Model file for the job. Use its own axes, mm. Face numbers are marked on the shaded views. A direction names the side the tool comes from. Round coordinates to 2 decimals unless told otherwise and drop trailing zeros. Loops run counter-clockwise (first coordinate to the right, second up) from the corner with the lowest first, then second, coordinate; pieces in that order, holes last. Notation, with made-up numbers: (-22.5, -25) -> (4.5, -25) arc R22 cw to (4.5, 2) -> close; hole circle Ø8 at (53, 79.5). An arc over 180 degrees is marked (long way). Use a Markdown table: item, result.
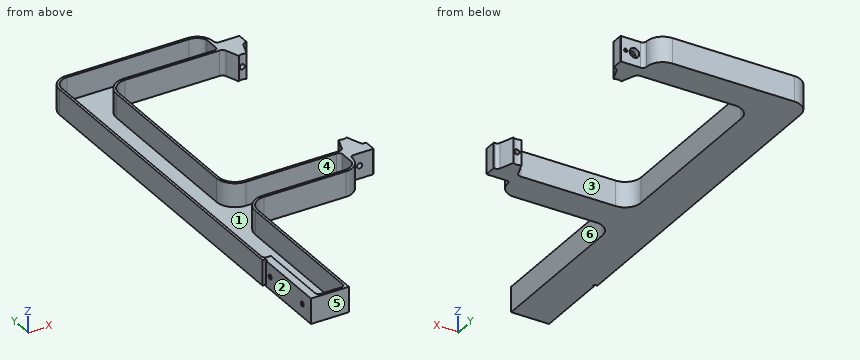
from build123d import *

# Parameters (mm, degrees)
BOSS_EXTRUDE1_DEPTH              = 15.875
SKETCH13_W                       = 2.54
SKETCH13_H                       = 95.25
CUT_EXTRUDE2_DEPTH               = 32.75
SKETCH14_W                       = 1.6002
SKETCH14_H                       = 3.302
CUT_EXTRUDE3_DEPTH               = 32.75
FILLET4_R                        = 1.5875
FILLET1_R                        = 6.35
FILLET2_R                        = 20
FILLET3_R                        = 4.7625
SKETCH10_R                       = 6
CUT_EXTRUDE1_DEPTH               = 7
F_4_40_TAPPED_HOLE1_D            = 2.2606
F_4_40_TAPPED_HOLE1_DEPTH        = 7.6
F_4_40_TAPPED_HOLE1_CSINK_D      = 4.1148
F_4_40_TAPPED_HOLE1_CSINK_ANGLE  = 90
F_4_40_TAPPED_HOLE1_TIP          = 0.679152758
CHAMFER1_SIZE                    = 0.5
F_10_32_TAPPED_HOLE1_D           = 4.0386
F_10_32_TAPPED_HOLE1_DEPTH       = 12.03
F_10_32_TAPPED_HOLE1_CSINK_D     = 6.096
F_10_32_TAPPED_HOLE1_CSINK_ANGLE = 90
F_10_32_TAPPED_HOLE1_TIP         = 1.213317848
CUT_EXTRUDE7_DEPTH               = 29.75
FILLET5_R                        = 4.7625


with BuildPart() as part:
    # Sketch1 → Boss-Extrude1 (new body, symmetric)
    with BuildSketch(Plane.XY):
        with BuildLine():
            Line((-313, -123), (-176.364963641, -123))
            Line((-176.364963641, -123), (-170.374987965, -123))
            Line((-170.374987965, -123), (-162.97678843, -102.673613833))
            ThreePointArc((-162.97678843, -102.673613833), (-158, -104), (-153.02321157, -102.673613833))
            Line((-153.02321157, -102.673613833), (-145.625012035, -123))
            Line((-145.625012035, -123), (-140.625012035, -123))
            Line((-140.625012035, -123), (-140.625012035, -138))
            Line((-140.625012035, -138), (-145.625012035, -138))
            Line((-145.625012035, -138), (-170.374987965, -138))
            Line((-170.374987965, -138), (-170.374987965, -163))
            Line((-170.374987965, -163), (-313, -163))
            Line((-313, -163), (-313, -370.4))
            Line((-313, -370.4), (-363, -370.4))
            Line((-363, -370.4), (-363, -163))
            Line((-363, -163), (-363, 163))
            Line((-363, 163), (-170.374987965, 163))
            Line((-170.374987965, 163), (-170.374987965, 138))
            Line((-170.374987965, 138), (-145.625012035, 138))
            Line((-145.625012035, 138), (-140.625012035, 138))
            Line((-140.625012035, 138), (-140.625012035, 123))
            Line((-140.625012035, 123), (-145.625012035, 123))
            Line((-145.625012035, 123), (-153.02321157, 102.673613833))
            ThreePointArc((-153.02321157, 102.673613833), (-158, 104), (-162.97678843, 102.673613833))
            Line((-162.97678843, 102.673613833), (-170.374987965, 123))
            Line((-170.374987965, 123), (-176.364963641, 123))
            Line((-176.364963641, 123), (-313, 123))
            Line((-313, 123), (-313, -123))
        make_face()
    extrude(amount=BOSS_EXTRUDE1_DEPTH, both=True)

    # Sketch13 → Cut-Extrude2 (cut, through all)
    with BuildSketch(Plane.XY.offset(15.875)):
        with Locations((-361.73, -322.775)):
            Rectangle(SKETCH13_W, SKETCH13_H)
    extrude(amount=-CUT_EXTRUDE2_DEPTH, mode=Mode.SUBTRACT)

    # Sketch14 → Cut-Extrude3 (cut, through all)
    with BuildSketch(Plane.XY.offset(15.875)):
        with Locations((-359.6599, -276.801)):
            Rectangle(SKETCH14_W, SKETCH14_H)
    extrude(amount=-CUT_EXTRUDE3_DEPTH, mode=Mode.SUBTRACT)

    # Fillet4
    fillet4_edges = [part.edges().sort_by_distance(p)[0] for p in [
        (-358.8598, -275.15, 0),
        (-358.8598, -278.452, 0),
    ]]
    fillet(fillet4_edges, radius=FILLET4_R)

    # Fillet1
    fillet1_edges = [part.edges().sort_by_distance(p)[0] for p in [
        (-170.374987965, -123, 0),
        (-170.374987965, 123, 0),
    ]]
    fillet(fillet1_edges, radius=FILLET1_R)

    # Fillet2
    fillet2_edges = [part.edges().sort_by_distance(p)[0] for p in [
        (-313, 123, 0),
        (-313, -123, 0),
        (-170.374987965, -163, 0),
        (-313, -163, 0),
        (-363, 163, 0),
        (-170.374987965, 163, 0),
    ]]
    fillet(fillet2_edges, radius=FILLET2_R)

    # Fillet3
    fillet3_edges = [part.edges().sort_by_distance(p)[0] for p in [
        (-145.625012035, -123, 0),
        (-170.374987965, -138, 0),
        (-170.374987965, 138, 0),
        (-145.625012035, 123, 0),
    ]]
    fillet(fillet3_edges, radius=FILLET3_R)

    # Sketch8 → M6 Clearance Hole1 (revolve, cut)
    with BuildSketch(Plane(origin=(-158, 138, 0), x_dir=(0, 0, 1), z_dir=(1, 0, 0))):
        Polygon((0, 0), (0, 51.960753981), (3.2, 50.038), (3.2, 0), align=None)
    m6_clearance_hole1 = revolve(axis=Axis((-158, 144.35, 0), (0, -1, 0)), mode=Mode.SUBTRACT)

    # Sketch10 → Cut-Extrude1 (cut)
    with BuildSketch(Plane(origin=(0, 138, 0), x_dir=(1, 0, 0), z_dir=(0, 1, 0))):
        with Locations(Location((-158, 0, 0), (0, 0, 270))):  # turned: the seam where the file's is
            Circle(SKETCH10_R)
    extrude(amount=-CUT_EXTRUDE1_DEPTH, mode=Mode.SUBTRACT)

    # #4-40 Tapped Hole1
    with Locations(Plane(origin=(0, 138, 0), x_dir=(-1, 0, 0), z_dir=(0, 1, 0))):
        with Locations((147, 0)):
            CounterSinkHole(F_4_40_TAPPED_HOLE1_D / 2, F_4_40_TAPPED_HOLE1_CSINK_D / 2, depth=F_4_40_TAPPED_HOLE1_DEPTH, counter_sink_angle=F_4_40_TAPPED_HOLE1_CSINK_ANGLE)
            with Locations((0, 0, -(F_4_40_TAPPED_HOLE1_DEPTH + F_4_40_TAPPED_HOLE1_TIP / 2))):  # 118° drill point
                Cone(0, F_4_40_TAPPED_HOLE1_D / 2, F_4_40_TAPPED_HOLE1_TIP, mode=Mode.SUBTRACT)

    # Mirror1: M6 Clearance Hole1 across plane
    add(m6_clearance_hole1.mirror(Plane.ZX), mode=Mode.SUBTRACT)

    # Chamfer1
    chamfer1_edges = [part.edges().sort_by_distance(p)[0] for p in [
        (-140.625012035, -138, 0),
        (-140.625012035, 138, 0),
    ]]
    chamfer(chamfer1_edges, length=CHAMFER1_SIZE)

    # #10-32 Tapped Hole1
    with Locations(Plane.ZY.offset(360.46)):
        with Locations((0, -286.58), (0, -352.62)):
            CounterSinkHole(F_10_32_TAPPED_HOLE1_D / 2, F_10_32_TAPPED_HOLE1_CSINK_D / 2, depth=F_10_32_TAPPED_HOLE1_DEPTH, counter_sink_angle=F_10_32_TAPPED_HOLE1_CSINK_ANGLE)
            with Locations((0, 0, -(F_10_32_TAPPED_HOLE1_DEPTH + F_10_32_TAPPED_HOLE1_TIP / 2))):  # 118° drill point
                Cone(0, F_10_32_TAPPED_HOLE1_D / 2, F_10_32_TAPPED_HOLE1_TIP, mode=Mode.SUBTRACT)

    # Sketch25 → Cut-Extrude7 (cut)
    with BuildSketch(Plane.XY.offset(15.875)):
        with BuildLine():
            Line((-190.374987965, 160), (-343, 160))
            ThreePointArc((-343, 160), (-355.02081528, 155.02081528), (-360, 143))
            Line((-360, 143), (-360, -272.15))
            Line((-360, -272.15), (-350.808, -272.15))
            Line((-350.808, -272.15), (-350.808, -367.4))
            Line((-350.808, -367.4), (-316, -367.4))
            Line((-316, -367.4), (-316, -183))
            ThreePointArc((-316, -183), (-309.263455967, -166.736544033), (-293, -160))
            Line((-293, -160), (-190.374987965, -160))
            ThreePointArc((-190.374987965, -160), (-181.091910782, -157.241645903), (-174.821305833, -149.861703296))
            Line((-174.821305833, -149.861703296), (-174.821305833, -126))
            Line((-174.821305833, -126), (-293, -126))
            ThreePointArc((-293, -126), (-309.263455967, -119.263455967), (-316, -103))
            Line((-316, -103), (-316, 103))
            ThreePointArc((-316, 103), (-309.263455967, 119.263455967), (-293, 126))
            Line((-293, 126), (-174.821305833, 126))
            Line((-174.821305833, 126), (-174.821305833, 149.861703296))
            ThreePointArc((-174.821305833, 149.861703296), (-181.091910782, 157.241645903), (-190.374987965, 160))
        make_face()
    extrude(amount=-CUT_EXTRUDE7_DEPTH, mode=Mode.SUBTRACT)

    # Fillet5
    fillet5_edges = [part.edges().sort_by_distance(p)[0] for p in [
        (-350.808, -367.4, 1),
        (-316, -367.4, 1),
        (-174.821305833, -149.861703296, 1),
        (-174.821305833, -126, 1),
        (-174.821305833, 126, 1),
        (-174.821305833, 149.861703296, 1),
        (-360, -272.15, 1),
    ]]
    fillet(fillet5_edges, radius=FILLET5_R)


solid = part.part
Q1. Pull direction Y, two halves, no side cores. Call the marked faces 4, 5 and 6: released by +Y, released by -Y, zero draft, split by the parting line, or undercut.
Results list:
| item | result |
|---|---|
| face 4 | undercut |
| face 5 | released by -Y |
| face 6 | zero draft |
Q2. Band-saw the part on C-C, the plane x = -329. Give the cut face in (y, z) (3 decimals), plus the area to 3 significant figures.
Results list:
| item | result |
|---|---|
| outline | (-370.4, -15.875) -> (163, -15.875) -> (163, 15.875) -> (160, 15.875) -> (160, -13.875) -> (-367.4, -13.875) -> (-367.4, 15.875) -> (-370.4, 15.875) -> close |
| area | 1,250 mm² |
Q3. Band-saw the part on B-B, the plane y = -69.5. Give the cut face in (x, z) (3 decimals), plus the area to 4 significant figures.
Results list:
| item | result |
|---|---|
| outline | (-363, -15.875) -> (-313, -15.875) -> (-313, 15.875) -> (-316, 15.875) -> (-316, -13.875) -> (-360, -13.875) -> (-360, 15.875) -> (-363, 15.875) -> close |
| area | 278.5 mm² |
Q4. Band-saw the part on A-A, the plane x = -196.5. Give the cut face in (y, z) (3 decimals).
Results list:
| item | result |
|---|---|
| outline | (-163, -15.875) -> (-123, -15.875) -> (-123, 15.875) -> (-126, 15.875) -> (-126, -13.875) -> (-160, -13.875) -> (-160, 15.875) -> (-163, 15.875) -> close; (123, -15.875) -> (163, -15.875) -> (163, 15.875) -> (160, 15.875) -> (160, -13.875) -> (126, -13.875) -> (126, 15.875) -> (123, 15.875) -> close |
Q5. Flat gauge pins, fed straight in: pin 1 (4 mm diameter, centred on x = -158, z = 0, fed in from +Y); pin 2 (12 mm diameter, centred on x = -157.5, z = 6, fed in from +Y); pin 3 (10 mm diameter, centred on y = 99, z = -4.5, fed in from +X); pin 4 (0.8 mm diameter, centred on x = -362, z = 6, fed in from -Y). Where does each tip first touch, or does it go through?
Results list:
| item | result |
|---|---|
| pin 1 | passes through |
| pin 2 | stops at y = 138 |
| pin 3 | stops at x = -152.54 |
| pin 4 | stops at y = -275.15 |
Q6. Tool access for the marked faces 1, 2 and 3: list every direction of +Z, -Z, +X, -X, +Y, -Y with a clear straight run to the whole face (end or side of a thin tool).
Results list:
| item | result |
|---|---|
| face 1 | +Z |
| face 2 | +Z, -Z, -X, -Y |
| face 3 | +Z, -Z |
Q7. Drill centre lines: L1, parallel to Y at x = -207.5, z = 12.5; L2, parallel to X at y = 134, z = 0; L3, parallel to Z at x = -147, y = 134.5 (3 decimals). Where is each one in solid material? Low to high. Write a range as from..to.
Results list:
| item | result |
|---|---|
| L1 | y = -163..-160, -126..-123, 123..126, 160..163 |
| L2 | x = -363..-360, -174.82..-164, -152..-148.13, -145.87..-140.63 |
| L3 | z = -15.875..-1.13, 1.13..15.875 |
